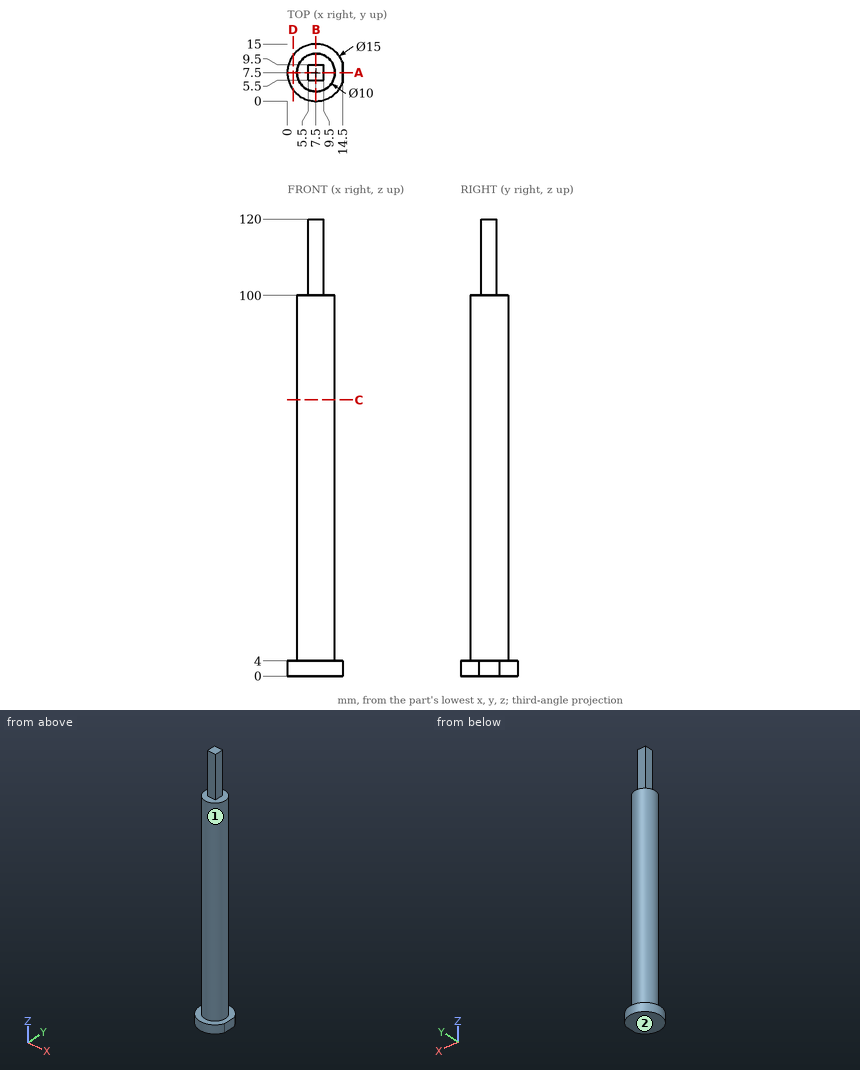
Study the drawing (mm; zero at the part's minimum x, y, z) and answer. A direction names the side the tool comes from. Give positions to 0.01 mm unless a question says otherwise; leave off trailing zeros. Loops run counter-clockwise (first coordinate to the right, second up) from the corner with the lowest first, then second, coordinate; pieces in that order, holes last. Notation, with made-up numbers: (-34, 33.25) - (-27, 33.25) arc R23 ccw to (-27, 55.25) - close; hole circle Ø11 at (-38, -21.75). An arc over 180 degrees is marked (long way). One line per question, with ' | ' between items.
(1) A tool of negligible diameter and unlimited length cuts with its end or side. For the marked faces 1 and 2, from which of +Z, -Z, +X, -X, +Y, -Y can it reach the whole face along a straight path? Write none if from no direction.
Recorded:
face 1: +Z | face 2: -Z, +X, -X, +Y, -Y
(2) The part is cut by section C-C (z = 72.5). Write down the section's boundary in (x, y), then the cut area to 3 significant figures.
Recorded:
outline: circle Ø10 at (7.5, 7.5) | area: 78.5 mm²
(3) The part is cut by section A-A (y = 7.5). Write down the section's boundary in (x, z).
Recorded:
outline: (0, 0) - (14.5, 0) - (14.5, 4) - (12.5, 4) - (12.5, 100) - (9.5, 100) - (9.5, 120) - (5.5, 120) - (5.5, 100) - (2.5, 100) - (2.5, 4) - (0, 4) - close
(4) Straight lines are drawn through the part: probe 1 along Z at (x, y) = (11.25, 11.5); probe 2 along Y at (x, z) = (7.5, 7.5); probe 3 along Y at (x, z) = (6.5, 115). For each, find the intervals that lie inside material, in ascending order.
Recorded:
probe 1: z = 0 to 4 | probe 2: y = 2.5 to 12.5 | probe 3: y = 5.5 to 9.5
(5) The part is cut by section B-B (x = 7.5). Write down the section's boundary in (y, z), then the cut area to 3 significant figures.
Recorded:
outline: (0, 0) - (15, 0) - (15, 4) - (12.5, 4) - (12.5, 100) - (9.5, 100) - (9.5, 120) - (5.5, 120) - (5.5, 100) - (2.5, 100) - (2.5, 4) - (0, 4) - close | area: 1,100 mm²
(6) The part is cut by section D-D (x = 1.5). Write down the section's boundary in (y, z), then the cut area to 3 significant figures.
Recorded:
outline: (3, 0) - (12, 0) - (12, 4) - (3, 4) - close | area: 36.0 mm²
(7) Each of these flat-tipped pins is pushed along its axis until it touches: pin 1 Ø1.2 at (x, z) = (8, 111.5) entering from -Y; pin 2 Ø2 at (y, z) = (8, 36) entering from +X; pin 3 Ø3 at (y, z) = (8, 111) entering from +X. Where does it stop, or does it pass through?
Recorded:
pin 1: stops at y = 5.5 | pin 2: stops at x = 12.5 | pin 3: stops at x = 9.5
